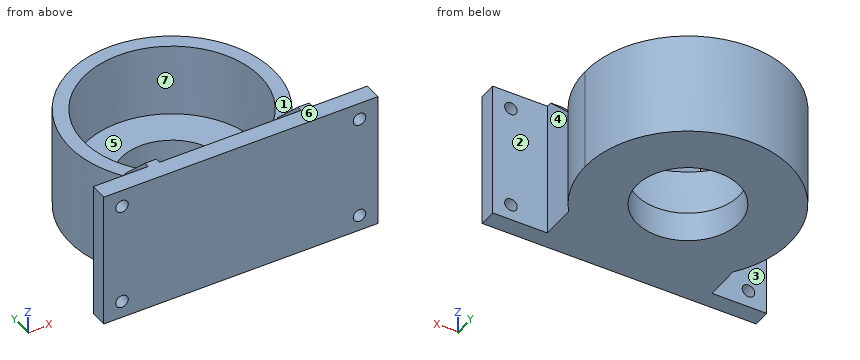
from build123d import *

# Parameters (mm, degrees)
F0_W      = 24
F0_H      = 7.6146386564
F1_DEPTH  = 45
F2_R      = 38.75
F4_DEPTH  = 32
F5_DEPTH  = 15
F7_DEPTH  = 15
F8_SIZE   = 14.99999
F9_R      = 2.75
F10_DEPTH = 25
F11_R     = 22.5
F12_DEPTH = 25


# Not quite as in the source:
# - a fillet or chamfer is up to 0.001 mm smaller than in the source, because OpenCascade refuses the exact size


with BuildPart() as f1:
    # F0 (on Top) → F1 (new body)
    with BuildSketch(Plane.XY):
        with BuildLine():
            ThreePointArc((36, -27), (42.6907484123, -14.2302494708), (45, 0))
            ThreePointArc((45, 0), (-14.2302494708, 42.6907484123), (-36, -27))
            Line((-36, -27), (36, -27))
        make_face()
        with BuildLine():
            ThreePointArc((-15.1652218257, -42.3676297069), (-26.7116265289, -36.2144861648), (-36, -27))
            Line((-36, -27), (-36, -42.3676297069))
            Line((-36, -42.3676297069), (-15.1652218257, -42.3676297069))
        make_face()
        with BuildLine():
            Line((36, -27), (-36, -27))
            ThreePointArc((-36, -27), (-26.7116265289, -36.2144861648), (-15.1652218257, -42.3676297069))
            Line((-15.1652218257, -42.3676297069), (15.1652218257, -42.3676297069))
            ThreePointArc((15.1652218257, -42.3676297069), (26.7116265289, -36.2144861648), (36, -27))
        make_face()
        with BuildLine():
            Line((15.1652218257, -42.3676297069), (-15.1652218257, -42.3676297069))
            ThreePointArc((-15.1652218257, -42.3676297069), (0, -45), (15.1652218257, -42.3676297069))
        make_face()
        with Locations((-48, -46.174949035)):
            Rectangle(F0_W, F0_H)
        with BuildLine():
            ThreePointArc((15.1652218257, -42.3676297069), (0, -45), (-15.1652218257, -42.3676297069))
            Line((-15.1652218257, -42.3676297069), (-36, -42.3676297069))
            Line((-36, -42.3676297069), (-36, -49.9822683632))
            Line((-36, -49.9822683632), (36, -49.9822683632))
            Line((36, -49.9822683632), (36, -42.3676297069))
            Line((36, -42.3676297069), (15.1652218257, -42.3676297069))
        make_face()
        with Locations((48, -46.174949035)):
            Rectangle(F0_W, F0_H)
        with BuildLine():
            Line((36, -42.3676297069), (36, -27))
            ThreePointArc((36, -27), (26.7116265289, -36.2144861648), (15.1652218257, -42.3676297069))
            Line((15.1652218257, -42.3676297069), (36, -42.3676297069))
        make_face()
    extrude(amount=F1_DEPTH)

    # F2 (on face) → F4 (cut)
    with BuildSketch(Plane.XY.offset(45)):
        Circle(F2_R)
    extrude(amount=-F4_DEPTH, mode=Mode.SUBTRACT)

    # F3 (on face) → F5 (join)
    with BuildSketch(Plane.XY.offset(45)):
        Polygon((-36, -42.3676297069), (-60, -42.3676297069), (-60, -49.9822683632), (60, -49.9822683632), (60, -42.3676297069), (36, -42.3676297069), align=None)
    extrude(amount=F5_DEPTH)

    # F6 (on face) → F7 (join)
    with BuildSketch(Plane.XY.offset(45)):
        Polygon((-31, -25.031657964), (-36, -25.031657964), (-36, -27), (-36, -42.3676297069), (-31, -42.3676297069), align=None)
        Polygon((36, -42.3676297069), (36, -27), (36, -25.031657964), (31, -25.031657964), (31, -42.3676297069), align=None)
    extrude(amount=F7_DEPTH)

    # F8 (size 15 in the source; OpenCascade refuses exactly that, so slightly less here)
    f8_edges = [f1.edges().sort_by_distance(p)[0] for p in [
        (-33.5, -25.031658, 60),
        (33.5, -25.031658, 60),
    ]]
    chamfer(f8_edges, length=F8_SIZE)

    # F9 (on face) → F10 (cut)
    with BuildSketch(Plane(origin=(0, -42.3676297069, 0), x_dir=(-1, 0, 0), z_dir=(0, 1, 0))):
        with Locations((52, 7.5)):
            Circle(F9_R)
        with Locations((52, 52.5)):
            Circle(F9_R)
        with Locations((-52, 7)):
            Circle(F9_R)
        with Locations((-52, 52.5)):
            Circle(F9_R)
    extrude(amount=-F10_DEPTH, mode=Mode.SUBTRACT)

    # F11 (on face) → F12 (cut)
    with BuildSketch(Plane.XY.offset(13)):
        Circle(F11_R)
    extrude(amount=-F12_DEPTH, mode=Mode.SUBTRACT)


solid = f1.part
Input: part model. Units: mm. Frame: model coordinates. Face numbers are marked on the shaded views. A direction names the side the tool comes from. Give positions to 0.01 mm unless a question says otherwise; leave off trailing zeros. Write each loop counter-clockwise with the first axis right and the second up, starting at its lowest first coordinate (ties: lowest second). Pieces come first, ordered by that corner, then holes.
Q1. First-contact query: P1, Ø5, axis at x = 12, z = 28.5, coming from the +Y side; P2, Ø12, axis at y = -7.5, z = 43.5, coming from the +X side (3 decimals); P3, Ø7, axis at x = -52, z = 7.5, coming from the +Y side. Flat tips, straight axial feed; report the tip coordinate or a pass-through.
Q2. Section B-B, the plane x = 52. Output: boundary loops of the cut face in (y, z), plus the area to 3 significant figures.
Q3. Section C-C, the plane x = -10. Output: boundary loops of the cut face in (y, z), plus the area to 3 significant figures.
Q4. Set-up query: the marked faces 1, 2 and 3. Return all of +Z, -Z, +X, -X, +Y, -Y with unobstructed straight access to the full face (end or side cutting, diameter ignored); none if empty.
Q5. Section A-A, the plane z = 32. Output: boundary loops of the cut face in (x, y), plus the area to 3 significant figures.
Q6. Material intervals for probe 1 along Z at (x, y) = (-52, -48); probe 2 along Z at (x, y) = (52, -47); probe 3 along Y at (x, z) = (-1.5, 16) (3 decimals), sorted ascending.
Q7. Section D-D, the plane z = 52.5. Output: boundary loops of the cut face in (x, y).
Q8. Pull-direction query (X, two-part tool) for the marked faces 4, 5, 6 and 7; classes: pulls with the +X half, pulls with the -X half, needs draft (parallel to the pull), parting line crosses it, or undercut.
Filled in:
1. P1: stops at y = 43.99
1. P2: stops at x = 44.975
1. P3: stops at y = -42.37
2. outline: (-49.98, 0) - (-42.37, 0) - (-42.37, 4.25) - (-49.98, 4.25) - close; (-49.98, 9.75) - (-42.37, 9.75) - (-42.37, 49.75) - (-49.98, 49.75) - close; (-49.98, 55.25) - (-42.37, 55.25) - (-42.37, 60) - (-49.98, 60) - close
2. area: 373 mm2
3. outline: (-49.98, 0) - (-20.16, 0) - (-20.16, 13) - (-37.44, 13) - (-37.44, 45) - (-42.37, 45) - (-42.37, 60) - (-49.98, 60) - close; (20.16, 0) - (43.87, 0) - (43.87, 45) - (37.44, 45) - (37.44, 13) - (20.16, 13) - close
3. area: 1,420 mm2
4. face 1: +Z, +Y
4. face 2: +Z, -Z, +X
4. face 3: +Z, -Z, -X
5. outline: (-60, -49.98) - (60, -49.98) - (60, -42.37) - (36, -42.37) - (36, -27) arc R45 ccw (long way) to (-36, -27) - (-36, -42.37) - (-60, -42.37) - close; hole circle Ø77.5 at (0, 0)
5. area: 2,760 mm2
6. probe 1: z = 0 to 4.75, 10.25 to 49.75, 55.25 to 60
6. probe 2: z = 0 to 4.25, 9.75 to 49.75, 55.25 to 60
6. probe 3: y = -49.982 to -38.721, 38.721 to 44.975
7. outline: (-60, -49.98) - (-54.75, -49.98) - (-54.75, -42.37) - (-60, -42.37) - close; (-49.25, -49.98) - (49.25, -49.98) - (49.25, -42.37) - (36, -42.37) - (36, -32.53) - (31, -32.53) - (31, -42.37) - (-31, -42.37) - (-31, -32.53) - (-36, -32.53) - (-36, -42.37) - (-49.25, -42.37) - close; (54.75, -49.98) - (60, -49.98) - (60, -42.37) - (54.75, -42.37) - close
8. face 4: pulls with the +X half
8. face 5: undercut
8. face 6: needs draft
8. face 7: undercut
